Study the drawing (mm; zero at the part's minimum x, y, z) and answer. A direction names the side the tool comes from. Round coordinates to 2 decimals unless told otherwise and drop trailing zeros. Write each loop counter-clockwise with the first axis right and the second up, starting at its lowest first coordinate (ties: lowest second). Pieces come first, ordered by that corner, then holes.
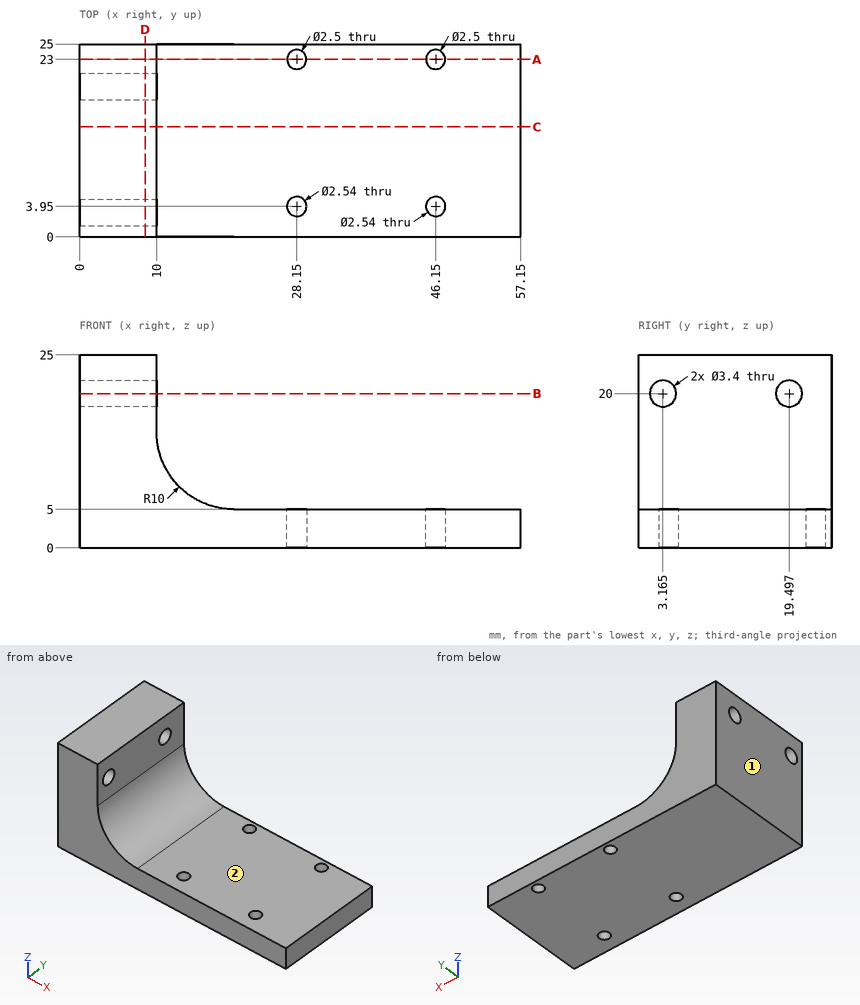
1. Section A-A on y = 23 is taken. Determine the outline of the cut face in (x, z), plus the area to 3 significant figures.
Geometry says:
outline: (0, 0) - (26.9, 0) - (26.9, 5) - (20, 5) arc R10 cw to (10, 15) - (10, 25) - (0, 25) - close; (29.4, 0) - (44.9, 0) - (44.9, 5) - (29.4, 5) - close; (47.4, 0) - (57.15, 0) - (57.15, 5) - (47.4, 5) - close
area: 482 mm2
2. Section C-C on y = 14.25 is taken. Determine the outline of the cut face in (x, z).
Geometry says:
outline: (0, 0) - (57.15, 0) - (57.15, 5) - (20, 5) arc R10 cw to (10, 15) - (10, 25) - (0, 25) - close
3. Section B-B on z = 20 is taken. Determine the outline of the cut face in (x, y) (3 decimals), plus the area to 3 significant figures.
Geometry says:
outline: (0, 0) - (10, 0) - (10, 1.465) - (0, 1.465) - close; (0, 4.865) - (10, 4.865) - (10, 17.797) - (0, 17.797) - close; (0, 21.197) - (10, 21.197) - (10, 25) - (0, 25) - close
area: 182 mm2
4. Straight lines are drawn through the part: line 1 along Y through (x, z) = (4.5, 20) (3 decimals); line 2 along Y through (x, z) = (28.15, 1.2); line 3 along X through (y, z) = (3.95, 3.15). For each, find the intervals that lie inside material, in ascending order.
Geometry says:
line 1: y = 0 to 1.465, 4.865 to 17.797, 21.197 to 25
line 2: y = 0 to 2.68, 5.22 to 21.75, 24.25 to 25
line 3: x = 0 to 26.88, 29.42 to 44.88, 47.42 to 57.15
5. Given pin 1 (12 mm diameter, centred on x = 23, y = 11, fed in from +Z); pin 2 (6 mm diameter, centred on x = 38.5, y = 3.5, fed in from +Z); pin 3 (6 mm diameter, centred on y = 4, z = 10, fed in from +X), each flat-ended and moving along its own axis, determine where each tip first touches the part or whether it passes through.
Geometry says:
pin 1: stops at z = 5.46
pin 2: stops at z = 5
pin 3: stops at x = 14
6. Section D-D on x = 8.5 is taken. Determine the outline of the cut face in (y, z) (3 decimals), plus the area to 3 significant figures.
Geometry says:
outline: (0, 0) - (25, 0) - (25, 25) - (0, 25) - close; hole circle Ø3.4 at (3.165, 20); hole circle Ø3.4 at (19.497, 20)
area: 607 mm2
7. A tool of negligible diameter and unlimited length cuts with its end or side. For the marked faces 1 and 2, from which of +Z, -Z, +X, -X, +Y, -Y can it reach the whole face along a straight path? Write none if from no direction.
Geometry says:
face 1: +Z, -Z, -X, +Y, -Y
face 2: +Z, +X, +Y, -Y
